Read the model definition and answer for the solid it produces. Units are mm, in the model's axes. A direction names the side the tool comes from. Round coordinates to 2 decimals unless told otherwise and drop trailing zeros. Write each loop counter-clockwise with the first axis right and the second up, starting at its lowest first coordinate (ties: lowest second). Pieces come first, ordered by that corner, then holes. Notation, with made-up numbers: (83, -3) - (124, -3) arc R21 ccw to (124, 12) - close; hole circle Ø2 at (-15, -14.75). An arc over 180 degrees is marked (long way). One line per item, written item: value. Start each with the question number.
(1) Find the intervals of material crossed by L1, parallel to Y at x = 0, z = 3.3; L2, parallel to Y at x = -15, z = 12.25; L3, parallel to X at y = -33.65, z = 2.25, in increasing order.
(2) The mould has two halves that part along Y. Classify faces 1 (the face through (-8.67, -39.05, 12.57)), 2 (the face through (36.94, -1.04, 2.46)), 3 (the face through (-1, 1, 25.5)): +Y half, -Y half, draft (parallel to the pull), parting line (faces both ways), or undercut.
(3) A cutting plane is placed at A-A, the plane y = 0. Determine the outline of the cut face in (x, z), plus the area to 3 significant figures.
(4) For faces 4 (the face through (-1, 1, 0)), 5 (the face through (0, -34, 5)), determine the directions among +Z, -Z, +X, -X, +Y, -Y from which every point of the face is accessible in a straight line to the end or side of a thin tool.
(5) A cutting plane is placed at D-D, the plane y = 33.65. Determine the outline of the cut face in (x, z), plus the area to 3 significant figures.
(6) A cutting plane is placed at C-C, the plane z = 16. Determine the outline of the cut face in (x, y), plus the area to 3 significant figures.
(7) Flat-ended cylindrical pins translate along their axes: pin 1 Ø10 at (y, z) = (-26.5, 15) entering from +X; pin 2 Ø2 at (x, z) = (24.5, 10) entering from -Y; pin 3 Ø3.5 at (x, y) = (-1, -33.5) entering from -Z. Find the tip coordinate at first contact, or state that the pin passes through.
from build123d import *

# Parameters (mm, degrees)
SKETCH1_R           = 40
BOSS_EXTRUDE1_DEPTH = 25.5
SKETCH2_R           = 3.45
CUT_EXTRUDE1_DEPTH  = 5


with BuildPart() as part:
    # Sketch1 → Boss-Extrude1 (new body)
    with BuildSketch(Plane.XY):
        Circle(SKETCH1_R)
    extrude(amount=BOSS_EXTRUDE1_DEPTH)

    # Sketch2 → Cut-Extrude1 (cut)
    with BuildSketch(Plane(origin=(0, 0, 0), x_dir=(-1, 0, 0), z_dir=(0, 0, -1))):
        with Locations((0, 33.65)):
            Circle(SKETCH2_R)
        with Locations((33.65, 0)):
            Circle(SKETCH2_R)
        with Locations(Location((0, -33.65, 0), (0, 0, 180))):
            Circle(SKETCH2_R)
        with Locations(Location((-33.65, 0, 0), (0, 0, 180))):
            Circle(SKETCH2_R)
    extrude(amount=-CUT_EXTRUDE1_DEPTH, mode=Mode.SUBTRACT)


solid = part.part
Here are the results:
1. L1: -40 to -37.1, -30.2 to 30.2, 37.1 to 40
1. L2: -37.08 to 37.08
1. L3: -21.63 to -3.45, 3.45 to 21.63
2. face 1: parting line
2. face 2: undercut
2. face 3: draft
3. outline: (-40, 0) - (-37.1, 0) - (-37.1, 5) - (-30.2, 5) - (-30.2, 0) - (30.2, 0) - (30.2, 5) - (37.1, 5) - (37.1, 0) - (40, 0) - (40, 25.5) - (-40, 25.5) - close
3. area: 1,970 mm²
4. face 4: -Z, +X, -X, +Y, -Y
4. face 5: -Z
5. outline: (-21.63, 0) - (-3.45, 0) - (-3.45, 5) - (3.45, 5) - (3.45, 0) - (21.63, 0) - (21.63, 25.5) - (-21.63, 25.5) - close
5. area: 1,070 mm²
6. outline: circle Ø80 at (0, 0)
6. area: 5,030 mm²
7. pin 1: x = 33.73
7. pin 2: y = -32.37
7. pin 3: z = 5
